from build123d import *

# Parameters (mm, degrees)
SKETCH1_W            = 117.3
SKETCH1_H            = 74
SKETCH1_W_2          = 114.3
SKETCH1_H_2          = 71
BOSS_EXTRUDE1_DEPTH  = 40.28
SKETCH5_W            = 117.3
SKETCH5_H            = 74
BOSS_EXTRUDE3_DEPTH  = 1.5
SKETCH7_W            = 69
SKETCH7_H            = 35.28
CUT_EXTRUDE3_DEPTH   = 2
SKETCH8_W            = 117.3
SKETCH8_H            = 74
BOSS_EXTRUDE4_DEPTH  = 1.5
SKETCH9_W            = 26
SKETCH9_H            = 3
BOSS_EXTRUDE5_DEPTH  = 6
SKETCH10_W           = 26
SKETCH10_H           = 2
BOSS_EXTRUDE6_DEPTH  = 11
SKETCH11_W           = 26
SKETCH11_H           = 2
BOSS_EXTRUDE7_DEPTH  = 3
SKETCH12_W           = 32
SKETCH12_H           = 6
BOSS_EXTRUDE8_DEPTH  = 1
SKETCH19_W           = 30
SKETCH19_H           = 32.28
CUT_EXTRUDE6_DEPTH   = 147.209193965
SKETCH20_W           = 55
SKETCH20_H           = 35
BOSS_EXTRUDE10_DEPTH = 13.5
SKETCH22_W           = 40
SKETCH22_H           = 3
CUT_EXTRUDE7_DEPTH   = 141.976481727


with BuildPart() as part:
    # Sketch1 → Boss-Extrude1 (new body)
    with BuildSketch(Plane(origin=(0, 0, 0), x_dir=(1, 0, 0), z_dir=(0, 1, 0))):
        with Locations((58.65, 37)):
            Rectangle(SKETCH1_W, SKETCH1_H)
        with Locations((58.65, 37)):
            Rectangle(SKETCH1_W_2, SKETCH1_H_2, mode=Mode.SUBTRACT)
    extrude(amount=BOSS_EXTRUDE1_DEPTH)

    # Sketch5 → Boss-Extrude3 (add)
    with BuildSketch(Plane.XZ):
        with Locations((58.65, -37)):
            Rectangle(SKETCH5_W, SKETCH5_H)
    extrude(amount=-BOSS_EXTRUDE3_DEPTH)

    # Sketch7 → Cut-Extrude3 (cut)
    with BuildSketch(Plane(origin=(117.3, 0, 0), x_dir=(0, 0, -1), z_dir=(1, 0, 0))):
        with Locations((37, 20.14)):
            Rectangle(SKETCH7_W, SKETCH7_H)
    extrude(amount=-CUT_EXTRUDE3_DEPTH, mode=Mode.SUBTRACT)

    # Sketch8 → Boss-Extrude4 (add)
    with BuildSketch(Plane(origin=(0, 40.28, 0), x_dir=(1, 0, 0), z_dir=(0, 1, 0))):
        with Locations((58.65, 37)):
            Rectangle(SKETCH8_W, SKETCH8_H)
    extrude(amount=-BOSS_EXTRUDE4_DEPTH)

    # Sketch9 → Boss-Extrude5 (add)
    with BuildSketch(Plane(origin=(0, 40.28, 0), x_dir=(1, 0, 0), z_dir=(0, 1, 0))):
        with Locations((14, 51.5)):
            Rectangle(SKETCH9_W, SKETCH9_H)
        with Locations((14, 22.5)):
            Rectangle(SKETCH9_W, SKETCH9_H)
    extrude(amount=BOSS_EXTRUDE5_DEPTH)

    # Sketch10 → Boss-Extrude6 (add)
    with BuildSketch(Plane.XY.offset(-50)):
        with Locations((14, 45.28)):
            Rectangle(SKETCH10_W, SKETCH10_H)
    extrude(amount=BOSS_EXTRUDE6_DEPTH)

    # Sketch11 → Boss-Extrude7 (add)
    with BuildSketch(Plane(origin=(0, 0, -24), x_dir=(-1, 0, 0), z_dir=(0, 0, -1))):
        with Locations((-14, 45.28)):
            Rectangle(SKETCH11_W, SKETCH11_H)
    extrude(amount=BOSS_EXTRUDE7_DEPTH)

    # Sketch12 → Boss-Extrude8 (add)
    with BuildSketch(Plane.ZY.offset(-1)):
        with Locations((-37, 43.28)):
            Rectangle(SKETCH12_W, SKETCH12_H)
    extrude(amount=BOSS_EXTRUDE8_DEPTH)

    # Sketch19 → Cut-Extrude6 (cut, through all)
    with BuildSketch(Plane.XY):
        with Locations((30, 20.14)):
            Rectangle(SKETCH19_W, SKETCH19_H)
        with Locations((87.3, 20.14)):
            Rectangle(SKETCH19_W, SKETCH19_H)
    extrude(amount=-CUT_EXTRUDE6_DEPTH, mode=Mode.SUBTRACT)

    # Sketch20 → Boss-Extrude10 (add)
    with BuildSketch(Plane.XZ.offset(-38.78)):
        with Locations((74.8, -37)):
            Rectangle(SKETCH20_W, SKETCH20_H)
    extrude(amount=BOSS_EXTRUDE10_DEPTH)

    # Sketch22 → Cut-Extrude7 (cut, through all)
    with BuildSketch(Plane.XZ.offset(-25.28)):
        with Locations((72.3, -24.5)):
            Rectangle(SKETCH22_W, SKETCH22_H)
        with Locations((72.3, -49.5)):
            Rectangle(SKETCH22_W, SKETCH22_H)
    extrude(amount=-CUT_EXTRUDE7_DEPTH, mode=Mode.SUBTRACT)


solid = part.part
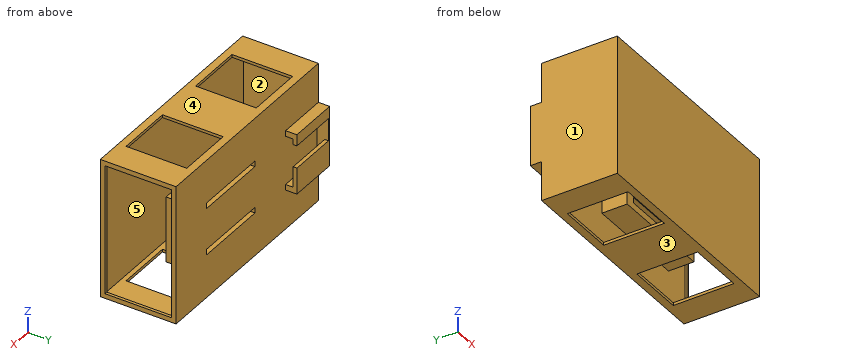
Part model, mm, in its own coordinate system. Face numbers are marked on the shaded views. A direction names the side the tool comes from. Coordinates: 2 decimals unless noted, no trailing zeros. Order: outer loops, then holes, each group sorted by start corner. A loop starts at its lowest first (then second) coordinate and runs counter-clockwise, first axis right, second up. Notation, with made-up numbers: M 12,20.5 L 38,20.5 A12 ccw 38,33.5 Z; hole C -21,-33.75 d1. An arc over 180 degrees is marked long. One line per question, with ' | ' between items.
Q1. Slice it at D-D (z = -36). Give the cut face in (x, y).
A:
outline: M 0,0 L 117.3,0 L 117.3,2.5 L 115.8,2.5 L 115.8,1.5 L 1.5,1.5 L 1.5,38.78 L 47.3,38.78 L 47.3,25.28 L 102.3,25.28 L 102.3,38.78 L 115.8,38.78 L 115.8,37.78 L 117.3,37.78 L 117.3,40.28 L 1,40.28 L 1,46.28 L 0,46.28 Z
Q2. 3-axis set-ups, long thin cutter, end or side, ignore diameter. For the marked faces 4 and 5: which of +Z, -Z, +X, -X, +Y, -Y reach the whole face in a straight line?
A:
face 4: +Z, +X, -X, +Y, -Y | face 5: none
Q3. Drill centre lines: line 1 (Y direction, x = 10.5, z = -49); line 2 (Z direction, x = 71, y = 31); line 3 (Y direction, x = 60, z = -55). Where is each one in solid material? Low to high.
A:
line 1: y = 0 to 1.5, 38.78 to 40.28, 44.28 to 46.28 | line 2: z = -74 to -72.5, -54.5 to -51, -48 to -26, -23 to -19.5, -1.5 to 0 | line 3: y = 0 to 1.5, 38.78 to 40.28
Q4. Pin check, flat tips, straight feed: P1, Ø6, axis at y = 16.5, z = -37.5, coming from the +X side; P2, Ø12, axis at x = 56.5, z = -55.5, coming from the +Y side; P3, Ø2.5, axis at y = 29.5, z = -49, coming from the +X side. Stop position of each tip, or through.
A:
P1: stops at x = 1.5 | P2: stops at y = 40.28 | P3: stops at x = 102.3
Q5. Slice it at B-B (y = 22.5). Give the cut face in (x, z).
A:
outline: M 0,-74 L 15,-74 L 15,-72.5 L 1.5,-72.5 L 1.5,-1.5 L 15,-1.5 L 15,0 L 0,0 Z; M 45,-74 L 72.3,-74 L 72.3,-72.5 L 45,-72.5 Z; M 45,-1.5 L 72.3,-1.5 L 72.3,0 L 45,0 Z; M 102.3,-74 L 117.3,-74 L 117.3,-71.5 L 115.8,-71.5 L 115.8,-72.5 L 102.3,-72.5 Z; M 102.3,-1.5 L 115.8,-1.5 L 115.8,-2.5 L 117.3,-2.5 L 117.3,0 L 102.3,0 Z
Q6. Two-plate mould, pull along X, no slides. Class the marked faces 1, 2 and 3: +X half, -X half, draft (parallel to the pull), parting line (faces both ways), or undercut.
A:
face 1: -X half | face 2: undercut | face 3: draft
Q7. Slice it at C-C (y = 28.5). Count the separate pieces of the cut face and the enclosed holes in it, and give its area (3 significant figures).
A:
separate pieces: 6 | enclosed holes: 2 | area: 1,970 mm^2
Q8. Slice it at A-A (x = 64). Give the cut face in (y, z).
A:
outline: M 0,-74 L 40.28,-74 L 40.28,-51 L 25.28,-51 L 25.28,-54.5 L 38.78,-54.5 L 38.78,-72.5 L 1.5,-72.5 L 1.5,-1.5 L 38.78,-1.5 L 38.78,-19.5 L 25.28,-19.5 L 25.28,-23 L 40.28,-23 L 40.28,0 L 0,0 Z; M 25.28,-48 L 40.28,-48 L 40.28,-26 L 25.28,-26 Z
